Check sheet for the drawn part. Datum: minimum x, y, z corner. Units: mm. A direction names the side the tool comes from. Give positions to 0.01 mm unless a question says otherwise; leave off trailing zeros. Order: outer loops, then holes, each group sorted by start corner. A loop starts at its lowest first (then second) coordinate and runs counter-clockwise, first axis right, second up.
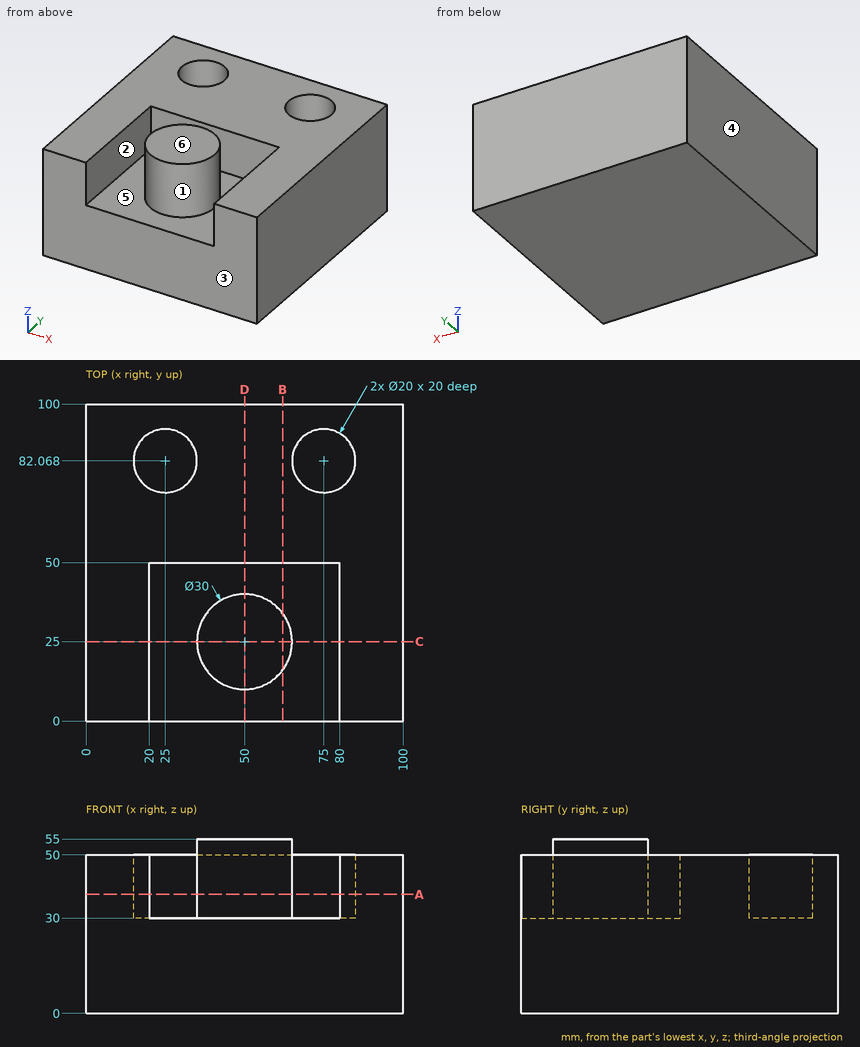
Q1. Go/stop test with flat-tipped pins: P1, Ø6, axis at x = 79, y = 86.5, coming from the +Z side; P2, Ø1, axis at x = 48.5, z = 35.5, coming from the -Y side; P3, Ø22, axis at x = 25, y = 83.5, coming from the +Z side. Record where each tip stops, or that it passes through.
Q2. Tool access check on the marked faces 5 and 6. Record the directions out of +Z, -Z, +X, -X, +Y, -Y that give a thin tool (end or side, any length) a straight path to the whole face; none if there is none.
Q3. Sectioned sample at B-B, the plane x = 62. Record the cut outline in (y, z), plus the area to 3 significant figures.
Q4. Sectioned sample at C-C, the plane y = 25. Record the cut outline in (x, z).
Q5. Material ranges on line 1 (Y direction, x = 25, z = 40); line 2 (X direction, y = 46.5, z = 44); line 3 (X direction, y = 76, z = 39.5), recorded low to high.
Q6. Sectioned sample at A-A, the plane z = 37.5. Record the cut outline in (x, y), plus the area to 3 significant figures.
Q7. Sectioned sample at D-D, the plane x = 50. Record the cut outline in (y, z), plus the area to 3 significant figures.
Q8. Draft check along X on the marked faces 1, 2, 3 and 4. Enter one of: pulls with the +X half, pulls with the -X half, needs draft (parallel to the pull), parting line crosses it, or undercut.
Filled in:
1. P1: stops at z = 30
1. P2: stops at y = 10.03
1. P3: stops at z = 50
2. face 5: +Z
2. face 6: +Z, +X, -X, +Y, -Y
3. outline: (0, 0) - (100, 0) - (100, 50) - (50, 50) - (50, 30) - (34, 30) - (34, 55) - (16, 55) - (16, 30) - (0, 30) - close
3. area: 4,450 mm2
4. outline: (0, 0) - (100, 0) - (100, 50) - (80, 50) - (80, 30) - (65, 30) - (65, 55) - (35, 55) - (35, 30) - (20, 30) - (20, 50) - (0, 50) - close
5. line 1: y = 50 to 72.07, 92.07 to 100
5. line 2: x = 0 to 20, 80 to 100
5. line 3: x = 0 to 17.05, 32.95 to 67.05, 82.95 to 100
6. outline: (0, 0) - (20, 0) - (20, 50) - (80, 50) - (80, 0) - (100, 0) - (100, 100) - (0, 100) - close; circle Ø30 at (50, 25); hole circle Ø20 at (25, 82.07); hole circle Ø20 at (75, 82.07)
6. area: 7,080 mm2
7. outline: (0, 0) - (100, 0) - (100, 50) - (50, 50) - (50, 30) - (40, 30) - (40, 55) - (10, 55) - (10, 30) - (0, 30) - close
7. area: 4,750 mm2
8. face 1: undercut
8. face 2: undercut
8. face 3: needs draft
8. face 4: pulls with the -X half
